Input: part model. Units: mm. Frame: model coordinates. Face numbers are marked on the shaded views. A direction names the side the tool comes from. Round coordinates to 2 decimals unless told otherwise and drop trailing zeros. Loops run counter-clockwise (first coordinate to the right, second up) from the corner with the lowest first, then second, coordinate; pieces in that order, holes last. Notation, with made-up numbers: (38.5, 81.25) -> (81.5, 81.25) arc R21 ccw to (81.5, 100.25) -> close; hole circle Ø3 at (-30, 41.25). An arc over 180 degrees is marked (long way). Answer in a Markdown table with one row per item. Add a question column.
Q1. Section C-C, the plane x = 32. Output: boundary loops of the cut face in (y, z), and give its area (3 significant figures).
Q2. Mould query, pull axis X, two halves, no side actions, for the marked faces 1, 2 and 3. Classes: pulls with the +X half, pulls with the -X half, needs draft (parallel to the pull), parting line crosses it, or undercut.
Q3. Section B-B, the plane y = 35. Output: boundary loops of the cut face in (x, z).
Q4. Section D-D, the plane z = 25. Output: boundary loops of the cut face in (x, y), and give its area (3 significant figures).
Q5. Reachability of the marked faces 4 and 5 from +Z, -Z, +X, -X, +Y, -Y: full face, straight path, thin tool, end or side. Return the list, or none.
Q6. Ray query, L1, parallel to Z at x = 20, y = 11.85; L2, parallel to X at y = 6, z = 30; L3, parallel to X at y = 13.1, z = 30. Return the intervals inside material, ascending. Write a range as from..to.
Q7. Pin query (flat end, axial travel): pin 1 (12 mm diameter, centred on x = 20, z = 30, fed in from -Y); pin 2 (3 mm diameter, centred on x = 44.5, z = 2.5, fed in from +Y); pin 3 (1 mm diameter, centred on x = 32.5, y = 17, fed in from +Z); pin 4 (11.5 mm diameter, centred on y = 35, z = 25, fed in from -X). Return the tip coordinate at first contact, or that it passes through.
Q8. Section A-A, the plane x = 90. Output: boundary loops of the cut face in (y, z).
```python
from build123d import *

# Parameters (mm, degrees)
IZIM1_W                     = 140
IZIM1_H                     = 50
Y_KSEKLIK_EKSTR_ZYON1_DEPTH = 60
IZIM2_W                     = 130
IZIM2_H                     = 50
KES_EKSTR_ZYON1_DEPTH       = 40
RADYUS1_R                   = 5
IZIM3_R                     = 15
IZIM3_R_2                   = 10
Y_KSEKLIK_EKSTR_ZYON2_DEPTH = 5
IZIM3_2_R                   = 10
KES_EKSTR_ZYON2_DEPTH       = 11
IZIM5_W                     = 70
IZIM5_H                     = 20
KES_EKSTR_ZYON3_DEPTH       = 11
IZIM6_W                     = 20
IZIM6_H                     = 40
KES_EKSTR_ZYON5_DEPTH       = 11
IZIM7_R                     = 10
KES_EKSTR_ZYON6_DEPTH       = 11
IZIM8_R                     = 5
KES_EKSTR_ZYON7_DEPTH       = 11


with BuildPart() as part:
    # Çizim1 → Yükseklik-Ekstrüzyon1 (new body)
    with BuildSketch(Plane.XY):
        with Locations((70, 25)):
            Rectangle(IZIM1_W, IZIM1_H)
    extrude(amount=Y_KSEKLIK_EKSTR_ZYON1_DEPTH)

    # Çizim2 → Kes-Ekstrüzyon1 (cut)
    with BuildSketch(Plane(origin=(0, 50, 0), x_dir=(1, 0, 0), z_dir=(0, 1, 0))):
        with Locations((65, -35)):
            Rectangle(IZIM2_W, IZIM2_H)
    extrude(amount=-KES_EKSTR_ZYON1_DEPTH, mode=Mode.SUBTRACT)

    # Radyus1
    radyus1_edges = [part.edges().sort_by_distance(p)[0] for p in [
        (130, 30, 10),
    ]]
    fillet(radyus1_edges, radius=RADYUS1_R)

    # Çizim3 → Yükseklik-Ekstrüzyon2 (add)
    with BuildSketch(Plane(origin=(0, 10, 0), x_dir=(1, 0, 0), z_dir=(0, 1, 0))):
        with Locations((20, -30)):
            Circle(IZIM3_R)
        with Locations((20, -30)):
            Circle(IZIM3_R_2, mode=Mode.SUBTRACT)
    extrude(amount=Y_KSEKLIK_EKSTR_ZYON2_DEPTH)

    # Çizim3<2> → Kes-Ekstrüzyon2 (cut, through all)
    with BuildSketch(Plane(origin=(0, 10, 0), x_dir=(1, 0, 0), z_dir=(0, 1, 0))):
        with Locations((20, -30)):
            Circle(IZIM3_2_R)
    extrude(amount=-KES_EKSTR_ZYON2_DEPTH, mode=Mode.SUBTRACT)

    # Çizim5 → Kes-Ekstrüzyon3 (cut, through all)
    with BuildSketch(Plane.XY.offset(10)):
        with Locations((35, 40)):
            Rectangle(IZIM5_W, IZIM5_H)
    extrude(amount=-KES_EKSTR_ZYON3_DEPTH, mode=Mode.SUBTRACT)

    # Çizim6 → Kes-Ekstrüzyon5 (cut, through all)
    with BuildSketch(Plane(origin=(0, 10, 0), x_dir=(1, 0, 0), z_dir=(0, 1, 0))):
        with Locations((60, -40)):
            Rectangle(IZIM6_W, IZIM6_H)
    extrude(amount=-KES_EKSTR_ZYON5_DEPTH, mode=Mode.SUBTRACT)

    # Çizim7 → Kes-Ekstrüzyon6 (cut, through all)
    with BuildSketch(Plane(origin=(0, 10, 0), x_dir=(1, 0, 0), z_dir=(0, 1, 0))):
        with Locations((90, -30)):
            Circle(IZIM7_R)
    extrude(amount=-KES_EKSTR_ZYON6_DEPTH, mode=Mode.SUBTRACT)

    # Çizim8 → Kes-Ekstrüzyon7 (cut, through all)
    with BuildSketch(Plane.ZY.offset(-130)):
        with Locations((25, 35)):
            Circle(IZIM8_R)
    extrude(amount=-KES_EKSTR_ZYON7_DEPTH, mode=Mode.SUBTRACT)


solid = part.part
```
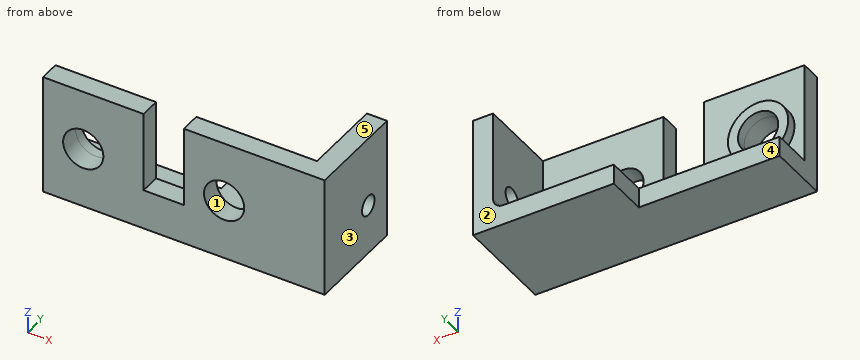
Answer block:
| question | item | result |
|---|---|---|
| 1 | outline | (0, 0) -> (30, 0) -> (30, 10) -> (10, 10) -> (10, 21) -> (15, 21) -> (15, 39) -> (10, 39) -> (10, 60) -> (0, 60) -> close |
| 1 | area | 890 mm^2 |
| 2 | face 1 | undercut |
| 2 | face 2 | needs draft |
| 2 | face 3 | pulls with the +X half |
| 3 | outline | (70, 0) -> (140, 0) -> (140, 20) -> (130, 20) -> (130, 15) arc R5 cw to (125, 10) -> (70, 10) -> close; (130, 30) -> (140, 30) -> (140, 60) -> (130, 60) -> close |
| 4 | outline | (0, 0) -> (11.34, 0) -> (11.34, 15) -> (5.86, 15) -> (5.86, 10) -> (0, 10) -> close; (28.66, 0) -> (50, 0) -> (50, 10) -> (34.14, 10) -> (34.14, 15) -> (28.66, 15) -> close; (70, 0) -> (81.34, 0) -> (81.34, 10) -> (70, 10) -> close; (98.66, 0) -> (140, 0) -> (140, 30) -> (130, 30) -> (130, 10) -> (98.66, 10) -> close; (130, 40) -> (140, 40) -> (140, 50) -> (130, 50) -> close |
| 4 | area | 1,210 mm^2 |
| 5 | face 4 | +Z, -Z, -X, +Y |
| 5 | face 5 | +Z, +X, -X, +Y, -Y |
| 6 | L1 | 0..10, 15..20, 40..45 |
| 6 | L2 | 0..10, 30..50, 70..80, 100..140 |
| 6 | L3 | 5..10, 30..35, 130..140 |
| 7 | pin 1 | through |
| 7 | pin 2 | y = 30 |
| 7 | pin 3 | z = 10 |
| 7 | pin 4 | x = 130 |
| 8 | outline | (0, 0) -> (50, 0) -> (50, 10) -> (10, 10) -> (10, 20) -> (0, 20) -> close; (0, 40) -> (10, 40) -> (10, 60) -> (0, 60) -> close |
